Design review of the part shown in the three views and the two pictorial views. Dimensions are in mm from the part's minimum x, y and z. A direction names the side the tool comes from. Round coordinates to 2 decimals unless told otherwise and drop trailing zeros. Loops run counter-clockwise (first coordinate to the right, second up) from the corner with the lowest first, then second, coordinate; pieces in that order, holes last.
1. Consider section B-B on y = 22.5. State the section outline as (x, z) points, then the cut area to 3 significant figures.
2. Tool access review of the marked faces 1 and 2: name each direction out of +Z, -Z, +X, -X, +Y, -Y from which nothing blocks a thin tool from reaching the whole face with its end or side.
3. To check wall thickness, follow line 1 along X through (y, z) = (63, 17); line 2 along Y through (x, z) = (17.5, 43); line 3 along Z through (x, y) = (2.5, 44.45). State the ranges of each line that lie inside material, in increasing order.
4. Consider section C-C on x = 98. State the section outline as (y, z) points.
5. Clearance check with flat-ended pins moving along their axes: pin 1 Ø15 at (y, z) = (44.45, 38.1) entering from -X; pin 2 Ø7 at (x, y) = (68, 4) entering from +Z. State where each tip first meets the part, or that it passes through.
6. Consider section D-D on y = 44.45. State the section outline as (x, z) points, then the cut area to 3 significant figures.
7. Draft analysis for pull direction X (two halves, no side actions). For the marked faces 3, 4 and 5, state which applies: released by +X, released by -X, zero draft, split by the parting line, or undercut.
8. Consider section A-A on z = 38.1. State the section outline as (x, y) points.
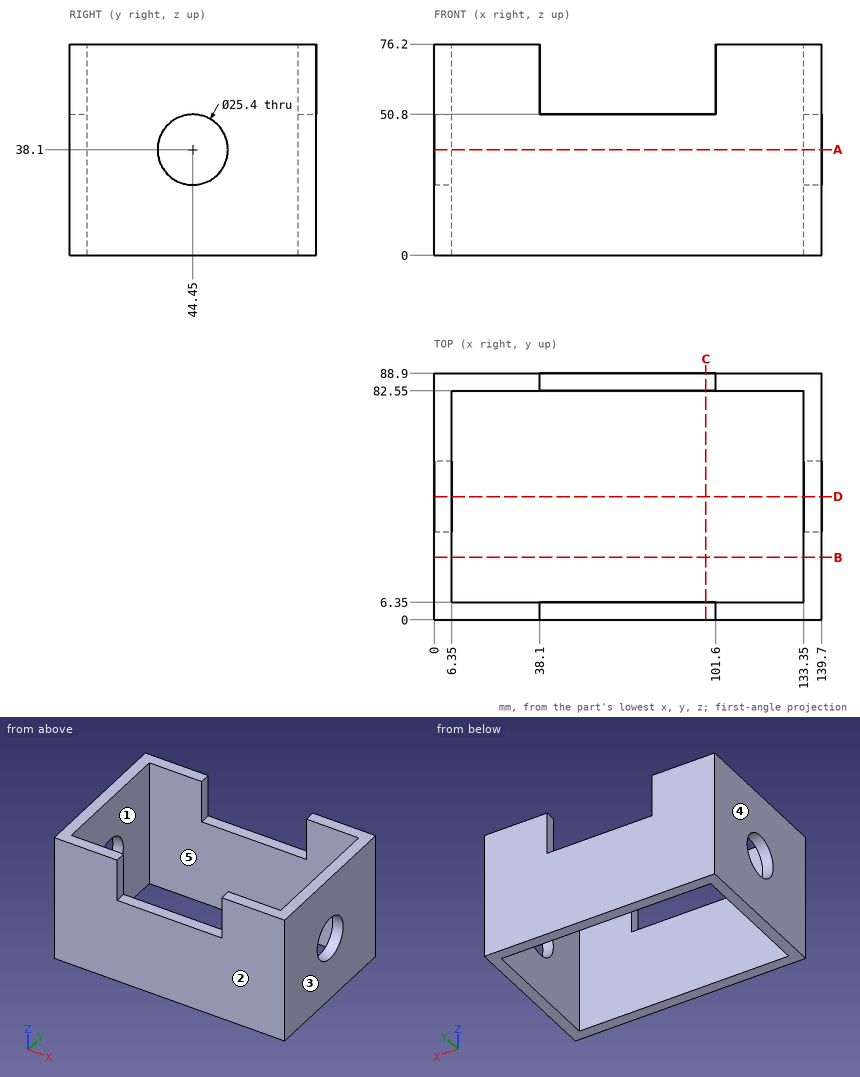
Resolved:
1. outline: (0, 0) - (6.35, 0) - (6.35, 76.2) - (0, 76.2) - close; (133.35, 0) - (139.7, 0) - (139.7, 76.2) - (133.35, 76.2) - close
1. area: 968 mm2
2. face 1: +Z, -Z
2. face 2: +Z, -Z, +X, -X, -Y
3. line 1: x = 0 to 6.35, 133.35 to 139.7
3. line 2: y = 0 to 6.35, 82.55 to 88.9
3. line 3: z = 0 to 25.4, 50.8 to 76.2
4. outline: (0, 0) - (6.35, 0) - (6.35, 50.8) - (0, 50.8) - close; (82.55, 0) - (88.9, 0) - (88.9, 50.8) - (82.55, 50.8) - close
5. pin 1: passes through
5. pin 2: stops at z = 50.8
6. outline: (0, 0) - (6.35, 0) - (6.35, 25.4) - (0, 25.4) - close; (0, 50.8) - (6.35, 50.8) - (6.35, 76.2) - (0, 76.2) - close; (133.35, 0) - (139.7, 0) - (139.7, 25.4) - (133.35, 25.4) - close; (133.35, 50.8) - (139.7, 50.8) - (139.7, 76.2) - (133.35, 76.2) - close
6. area: 645 mm2
7. face 3: released by +X
7. face 4: released by -X
7. face 5: undercut
8. outline: (0, 0) - (139.7, 0) - (139.7, 31.75) - (133.35, 31.75) - (133.35, 6.35) - (6.35, 6.35) - (6.35, 31.75) - (0, 31.75) - close; (0, 57.15) - (6.35, 57.15) - (6.35, 82.55) - (133.35, 82.55) - (133.35, 57.15) - (139.7, 57.15) - (139.7, 88.9) - (0, 88.9) - close
